Autodesk Inventor part; units mm, degrees
ref_plane "YZ Plane" through (0, 0, 0) normal (1, 0, 0) x (0, 1, 0)
ref_plane "XZ Plane" through (0, 0, 0) normal (0, 1, 0) x (-1, 0, 0)
ref_plane "XY Plane" through (0, 0, 0) normal (0, 0, 1) x (1, 0, 0)
sketch "Sketch1" plane through (0, 0, 0) normal (0, 1, 0) x (-1, 0, 0)
  line L0 (0, 0) -> (-30, 0)
  line L1 (-30, 0) -> (-30, 30)
  line L2 (-30, 30) -> (0, 30)
  line L3 (0, 30) -> (0, 0)
  line L4 (-2, 28) -> (-28, 28)
  line L5 (-28, 28) -> (-28, 2)
  line L6 (-28, 2) -> (-2, 2)
  line L7 (-2, 2) -> (-2, 28)
  line L8 (-10, 0) -> (-20, 0)
  line L9 (-20, 0) -> (-20, 30)
  line L10 (-20, 30) -> (-10, 30)
  line L11 (-10, 30) -> (-10, 0)
  line L12 (-10, 0) -> (-20, 30) construction
  line L13 (-20, 0) -> (-10, 30) construction
  point P0 (-15, 15)
  point P1 (-20, 2)
  point P2 (-10, 2)
  dimension "d0" = 30
  dimension "d1" = 30
  dimension "d2" = 2
  dimension "d3" = 10
  dimension "d4" = 30
  dimension "d5" = 15
extrude "Extrusion1" add sketch "Sketch1" along normal blind 2560 contours L0 L11 L6 L7 L4 L2 L3 | L0 L1 L2 L9 L4 L5 L6 | L11 L4 L9 L2
sketch "Sketch2" plane through (20, 0, 0) normal (0, 0, -1) x (-1, 0, 0)
  line L0 (-10, 0) -> (0, 0)
  line L1 (0, 0) -> (0, 2560)
  line L2 (-10, 2560) -> (0, 2560)
  line L3 (-10, 0) -> (-10, 2560)
  line L4 (10, 0) -> (20, 0)
  line L5 (20, 0) -> (20, 2560)
  line L6 (10, 2560) -> (20, 2560)
  line L7 (10, 0) -> (10, 2560)
  line L8 (-8, 2560) -> (18, 2560) construction
  line L9 (5, 2560) -> (5, 2050) construction
  circle A0 centre (5, 2050) radius 7.5
  line L10 (-8, 0) -> (18, 0) construction
  line L11 (5, 0) -> (5, 510) construction
  circle A1 centre (5, 510) radius 7.5
  point P0 (10, 2055.5902)
  point P1 (10, 2044.4098)
  point P2 (0, 2055.5902)
  point P3 (0, 2044.4098)
  point P4 (10, 515.5902)
  point P5 (10, 504.4098)
  point P6 (0, 515.5902)
  point P7 (0, 504.4098)
  dimension "d8" = 510
  dimension "d9" = 15
  dimension "d10" = 510
  dimension "d11" = 15
extrude "Extrusion2" cut sketch "Sketch2" against normal up to surface (2 mm away) contours A1 L1 | L7 A1 | L1 A0 | A0 L7
equation "\"d4\" = d1"
equation "\"d10\" = d8"
properties part number "guiaPorta"
Input: part model. Units: mm. Frame: model coordinates. Coordinates: 2 decimals unless noted, no trailing zeros. Write each loop counter-clockwise with the first axis right and the second up, starting at its lowest first coordinate (ties: lowest second). Pieces come first, ordered by that corner, then holes. Notation, with made-up numbers: M -31,77 L 4,77 A29 ccw 4,102 Z; hole C -6,-34.5 d2. An arc over 180 degrees is marked long. Use one line per item in the form item = value.
Q1. Material intervals for probe 1 along X at (y, z) = (1275.5, 23.5); probe 2 along Z at (x, y) = (18.5, 2121.5), sorted ascending. Write a range as from..to.
Answer below:
probe_1 = 0..2, 28..30
probe_2 = 28..30
Q2. Section A-A (z = 6.75). Return loops of the section in (x, y).
Answer below:
outline = M 0,0 L 2,0 L 2,2560 L 0,2560 Z; M 28,0 L 30,0 L 30,2560 L 28,2560 Z
Q3. Section B-B (y = 1507.5). Return loops of the section in (x, z).
Answer below:
outline = M 0,0 L 10,0 L 10,2 L 2,2 L 2,28 L 28,28 L 28,2 L 20,2 L 20,0 L 30,0 L 30,30 L 0,30 Z
